Autodesk Fusion 360 part; units mm, degrees
sketch "Sketch1" plane through (0, 0, 0) normal (0, 1, 0) x (1, 0, 0)
  line L0 (0, 0) -> (35, -80)
  line L1 (35, -80) -> (65, -80)
  line L2 (65, -80) -> (100, 0)
  line L3 (100, 0) -> (0, 0)
  circle A0 centre (50, -50) radius 7.5
  circle A1 centre (50, -50) radius 3
  dimension "d1" = 100
  dimension "d2" = 30
  dimension "d4" = 80
  dimension "d5" = 35
  dimension "d6" = 50
  dimension "d7" = 15
  dimension "d8" = 15
  dimension "d13" = 6
extrude "Extrude1" add sketch "Sketch1" against normal blind 5 contours L0 L1 L2 L3 | A0 | A1
extrude "Extrude2" add sketch "Sketch1" along normal blind 34 contours A1
fillet "Fillet1" radius 9 2 edges at (65, -2.5, 80) (35, -2.5, 80)
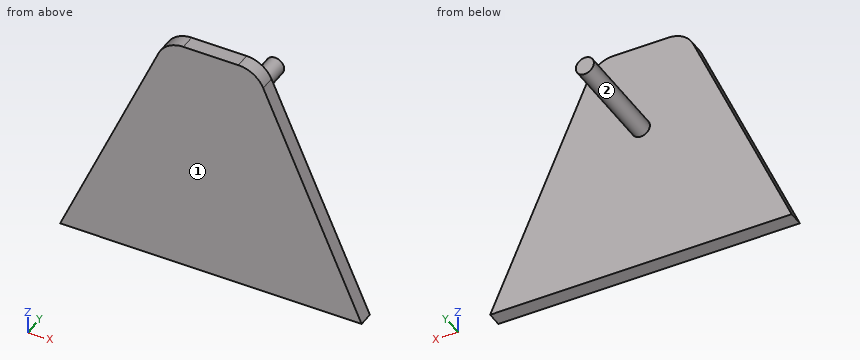
The listing builds one solid part. Answer for the finished solid, in the listing's coordinates (mm). Face numbers are marked on the shaded views. A direction names the side the tool comes from. Coordinates: 2 decimals unless noted, no trailing zeros. Order: outer loops, then holes, each group sorted by start corner. A loop starts at its lowest first (then second) coordinate and runs counter-clockwise, first axis right, second up. Notation, with made-up numbers: (44.25, -5) -> (72.25, -5) arc R19 cw to (72.25, -1) -> close; hole circle Ø9 at (-19.5, 36). An arc over 180 degrees is marked (long way). Answer in a Markdown table with one row per item. Add a question column.
Item 1: Which of the six approach directions +Z, -Z, +X, -X, +Y, -Y give full straight-line access (tool end or side, diameter ignored) to the marked faces 1 and 2?
Item 2: Find section C-C (y = 27.5). Write down the section's boundary in (x, z).
Item 3: Find section B-B (z = 50). Write down the section's boundary in (x, y) (3 decimals).
Item 4: Find section A-A (x = 50). Write down the section's boundary in (y, z).
Item 5: Find the intervals of material crossed by L1, parallel to Y at x = 74.5, z = 40.5; L2, parallel to X at y = -1.5, z = 62 (3 decimals); L3, parallel to X at y = 9, z = 51.5, in increasing order. Write a range as from..to.
Item 6: Find section D-D (x = 93). Write down the section's boundary in (y, z).
Item 7: Each of these flat-tipped pins is pushed along its axis until it touches: P1, Ø1.5, axis at x = 51, y = 3, coming from the -Z side; P2, Ø12, axis at y = 7.5, z = 33, coming from the +X side. Where does it stop, or does it pass through?
Result set:
| question | item | result |
|---|---|---|
| 1 | face 1 | +Z, -Z, +X, -X, -Y |
| 1 | face 2 | +Y |
| 2 | outline | circle Ø6 at (50, 50) |
| 3 | outline | (21.875, -5) -> (78.125, -5) -> (78.125, 0) -> (53, 0) -> (53, 34) -> (47, 34) -> (47, 0) -> (21.875, 0) -> close |
| 4 | outline | (-5, 0) -> (0, 0) -> (0, 47) -> (34, 47) -> (34, 53) -> (0, 53) -> (0, 80) -> (-5, 80) -> close |
| 5 | L1 | y = -5..0 |
| 5 | L2 | x = 27.125..72.875 |
| 5 | L3 | x = 47.4..52.6 |
| 6 | outline | (-5, 0) -> (0, 0) -> (0, 16) -> (-5, 16) -> close |
| 7 | P1 | stops at z = 47.01 |
| 7 | P2 | passes through |
